Here's how the part is built. I have some questions about the finished solid (model axes, mm). Round coordinates to 2 decimals unless told otherwise and drop trailing zeros. Order: outer loops, then holes, each group sorted by start corner. A loop starts at its lowest first (then second) coordinate and runs counter-clockwise, first axis right, second up. Notation, with made-up numbers: (-10.5, 49.25) - (26.5, 49.25) arc R16 ccw to (26.5, 60.25) - close; hole circle Ø6 at (58.25, 2). An arc over 180 degrees is marked (long way). Answer as a JSON object with one key per item and string values.
Autodesk Inventor part; units mm, degrees
ref_plane "YZ Plane" through (0, 0, 0) normal (1, 0, 0) x (0, 1, 0)
ref_plane "XZ Plane" through (0, 0, 0) normal (0, 1, 0) x (-1, 0, 0)
ref_plane "XY Plane" through (0, 0, 0) normal (0, 0, 1) x (1, 0, 0)
sketch "Sketch1" plane through (0, 0, 0) normal (0, 1, 0) x (-1, 0, 0)
  line L0 (-127.7724, 127.5062) -> (122.2276, 127.5062)
  line L1 (122.2276, 127.5062) -> (122.2276, -122.4938)
  line L2 (122.2276, -122.4938) -> (-127.7724, -122.4938)
  line L3 (-127.7724, -122.4938) -> (-127.7724, 127.5062)
  line L4 (104.2276, -104.4938) -> (104.2276, 109.5062)
  line L5 (104.2276, -104.4938) -> (-109.7724, -104.4938)
  line L6 (-109.7724, -104.4938) -> (104.2276, -104.4938)
  line L7 (122.2276, 109.5062) -> (122.2276, 88.1062)
  line L8 (122.2276, 88.1062) -> (104.2276, 88.1062)
  line L9 (104.2276, 88.1062) -> (104.2276, 109.5062)
  line L10 (122.2276, 45.3062) -> (104.2276, 45.3062)
  line L11 (104.2276, 45.3062) -> (104.2276, 23.9062)
  line L12 (104.2276, 23.9062) -> (122.2276, 23.9062)
  line L13 (104.2276, -18.8938) -> (122.2276, -18.8938)
  line L14 (122.2276, -40.2938) -> (104.2276, -40.2938)
  line L15 (122.2276, -83.0938) -> (104.2276, -83.0938)
  line L16 (-127.7724, 127.5062) -> (-127.7724, 109.5062)
  line L17 (104.2276, 109.5062) -> (104.2276, 127.5062)
  line L18 (-127.7724, -83.0938) -> (-109.7724, -83.0938)
  line L19 (-127.7724, -40.2938) -> (-109.7724, -40.2938)
  line L20 (-109.7724, -18.8938) -> (-127.7724, -18.8938)
  line L21 (-109.7724, 23.9062) -> (-127.7724, 23.9062)
  line L22 (-127.7724, 45.3062) -> (-109.7724, 45.3062)
  line L23 (-127.7724, 88.1062) -> (-109.7724, 88.1062)
  line L24 (18.6276, -104.4938) -> (18.6276, -122.4938)
  line L25 (-24.1724, -104.4938) -> (-24.1724, -122.4938)
  line L26 (-45.5724, -122.4938) -> (-45.5724, -104.4938)
  line L27 (-88.3724, -122.4938) -> (-88.3724, -104.4938)
  line L28 (40.0276, -122.4938) -> (40.0276, -104.4938)
  line L29 (82.8276, -122.4938) -> (82.8276, -104.4938)
  line L30 (18.6276, 127.5062) -> (18.6276, 109.5062)
  line L31 (40.0276, 109.5062) -> (40.0276, 127.5062)
  line L32 (82.8276, 109.5062) -> (82.8276, 127.5062)
  line L33 (-45.5724, 109.5062) -> (-45.5724, 127.5062)
  line L34 (-88.3724, 109.5062) -> (-88.3724, 127.5062)
  line L35 (-24.1724, 127.5062) -> (-24.1724, 109.5062)
  line L36 (104.2276, 109.5062) -> (-109.7724, 109.5062)
  line L37 (-109.7724, 109.5062) -> (-109.7724, -104.4938)
  line L38 (-109.7724, 109.5062) -> (-127.7724, 109.5062)
  line L39 (-127.7724, 109.5062) -> (-127.7724, 127.5062)
  line L40 (-127.7724, 127.5062) -> (-109.7724, 127.5062)
  line L41 (-109.7724, 127.5062) -> (-109.7724, 109.5062)
  line L42 (-109.7724, -104.4938) -> (-127.7724, -104.4938)
  line L43 (-127.7724, -104.4938) -> (-127.7724, -122.4938)
  line L44 (-127.7724, -122.4938) -> (-109.7724, -122.4938)
  line L45 (-109.7724, -122.4938) -> (-109.7724, -104.4938)
  line L46 (104.2276, -104.4938) -> (122.2276, -104.4938)
  line L47 (122.2276, -104.4938) -> (122.2276, -122.4938)
  line L48 (122.2276, -122.4938) -> (104.2276, -122.4938)
  line L49 (104.2276, -122.4938) -> (104.2276, -104.4938)
  line L50 (104.2276, 109.5062) -> (122.2276, 109.5062)
  line L51 (122.2276, 109.5062) -> (122.2276, 127.5062)
  line L52 (122.2276, 127.5062) -> (104.2276, 127.5062)
  line L53 (104.2276, 127.5062) -> (104.2276, 109.5062)
  point P0 (0, 0)
  point P1 (-127.7724, -18.8938)
  point P2 (-109.7724, -104.4938)
  point P3 (-109.7724, -104.4938)
  dimension "d0" = 250
  dimension "d1" = 250
  dimension "d2" = 21.4
extrude "Plate1" add sketch "Sketch1" along normal blind 18 contours L38 L37 L23 L3 | L0 L33 L36 L34 | L36 L4 L5 L37 | L22 L37 L21 L3 | L0 L30 L36 L35 | L20 L37 L19 L3 | L0 L32 L36 L31 | L18 L37 L42 L3 | L50 L1 L8 L4 | L5 L26 L2 L27 | L10 L1 L12 L4 | L5 L24 L2 L25 | L13 L1 L14 L4 | L5 L29 L2 L28 | L15 L1 L46 L4
sketch "Sketch2" plane through (0, 18, 0) normal (0, 1, 0) x (1, 0, 0)
  circle A0 centre (0, 0) radius 77.1
  line L0 (-65, 65) -> (65, 65)
  line L1 (65, 65) -> (65, -65)
  line L2 (65, -65) -> (-65, -65)
  line L3 (-65, -65) -> (-65, 65)
  line L4 (-65, 65) -> (65, -65) construction
  line L5 (65, 65) -> (-65, -65) construction
  circle A1 centre (65, 65) radius 1.5
  circle A2 centre (65, -65) radius 1.5
  circle A3 centre (-65, -65) radius 1.5
  circle A4 centre (-65, 65) radius 1.5
  dimension "d4" = 154.2
  dimension "d5" = 130
  dimension "d6" = 130
  dimension "d7" = 3
  dimension "d8" = 3
  dimension "d9" = 3
  dimension "d10" = 3
extrude "Cut1" cut sketch "Sketch2" against normal blind 18 contours A0 L1 | L1 A0 L2 L3 L0 | L0 A0 | A1 L0 L1 | L1 L0 A1 | A0 L2 | A2 L2 L1 | L1 L2 A2 | L3 A0 | A4 L3 L0 | L0 L3 A4 | A3 L3 L2 | L2 L3 A3
equation "\"d11\" = Thickness"
equation "\"d3\" = Thickness"
equation "\"BendRadius\" = Thickness"
equation "\"BendReliefWidth\" = Thickness"
equation "\"BendReliefDepth\" = 0.5 * Thickness"
equation "\"CornerReliefSize\" = 4 * Thickness"
equation "\"MinimumRemnant\" = 2 * Thickness"
equation "\"TransitionRadius\" = BendRadius"
equation "\"JacobiRadiusSize\" = BendRadius"
equation "\"GapSize\" = Thickness"
properties part number "2"
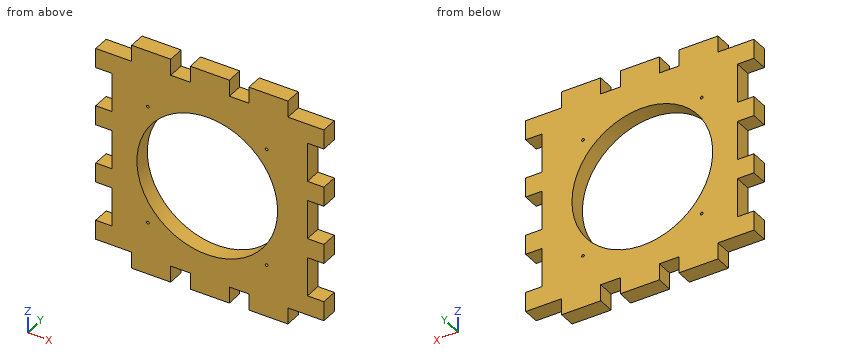
1. Imagine slicing it at C-C (y = 5.5). Give the number of separate pieces and of enclosed holes in the cut face, plus the area to 3 significant figures.
Responses:
{"separate pieces": "1", "enclosed holes": "5", "area": "34,800 mm2"}
2. Imagine slicing it at B-B (x = -50.5). List the corners of the cut face in (y, z) for me, plus the area to 3 significant figures.
Responses:
{"outline": "(0, -122.49) - (18, -122.49) - (18, -58.26) - (0, -58.26) - close; (0, 58.26) - (18, 58.26) - (18, 127.51) - (0, 127.51) - close", "area": "2,400 mm2"}
3. If I drill on L1, parallel to X at y = 8.25, z = 0; L2, parallel to Z at x = 65, y = 12.25; L3, parallel to Z at x = 0, y = 5.25, over which ranges is the centre line in solid material (lowest first)? Write a range as [from, to].
Responses:
{"L1": "[-104.23, -77.1], [77.1, 109.77]", "L2": "[-122.49, -66.5], [-63.5, -41.47], [41.47, 63.5], [66.5, 127.51]", "L3": "[-122.49, -77.1], [77.1, 127.51]"}
4. Imagine slicing it at A-A (z = 0). List the corners of the cut face in (x, y) for me.
Responses:
{"outline": "(-104.23, 0) - (-77.1, 0) - (-77.1, 18) - (-104.23, 18) - close; (77.1, 0) - (109.77, 0) - (109.77, 18) - (77.1, 18) - close"}
5. For P1, Ø2, axis at y = 15.5, z = -14, coming from the +X side; P2, Ø2, axis at x = 25.5, y = 15, coming from the +Z side; P3, Ø5.5, axis at x = 116, y = 6, coming from the -Z side; P4, Ø5, axis at x = 44.5, z = -97, coming from the -Y side, each with a flat end and sliding along its axis, tell me the tip position at first contact or that it passes through.
Responses:
{"P1": "x = 109.77", "P2": "z = 109.51", "P3": "z = -104.49", "P4": "y = 0"}
6. Imagine slicing it at D-D (x = 100). List the corners of the cut face in (y, z) for me, plus the area to 3 significant figures.
Responses:
{"outline": "(0, -104.49) - (18, -104.49) - (18, 109.51) - (0, 109.51) - close", "area": "3,850 mm2"}
